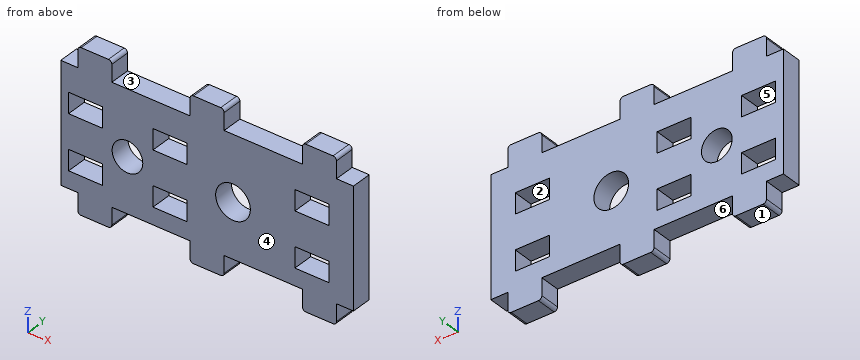
```python
from build123d import *

# Parameters (mm, degrees)
SKETCH1_W               = 86
SKETCH1_H               = 35
BOSS_EXTRUDE1_DEPTH     = 6
SKETCH2_R               = 5.1
SKETCH2_R_2             = 4.5
CUT_EXTRUDE1_DEPTH      = 6
SKETCH234_W             = 10
SKETCH234_H             = 6
BOSS_EXTRUDE234_DEPTH   = 6
FILLET134_R             = 1
SKETCH2341_W            = 10
SKETCH2341_H            = 6
BOSS_EXTRUDE2341_DEPTH  = 6
FILLET1341_R            = 1
SKETCH2342_W            = 10
SKETCH2342_H            = 6
BOSS_EXTRUDE2342_DEPTH  = 6
FILLET1342_R            = 1
FILLET134_OF_MIRROR1_R  = 1
FILLET1341_OF_MIRROR1_R = 1
FILLET1342_OF_MIRROR1_R = 1
SKETCH6_W               = 10
SKETCH6_H               = 6
CUT_EXTRUDE11_DEPTH     = 4
SKETCH61_W              = 10
SKETCH61_H              = 6
CUT_EXTRUDE12_DEPTH     = 4
SKETCH62_W              = 10
SKETCH62_H              = 6
CUT_EXTRUDE13_DEPTH     = 4


with BuildPart() as part:
    # Sketch1 → Boss-Extrude1 (new body)
    with BuildSketch(Plane(origin=(0, 0, 0), x_dir=(1, 0, 0), z_dir=(0, 1, 0))):
        with Locations((43, 17.5)):
            Rectangle(SKETCH1_W, SKETCH1_H)
    extrude(amount=BOSS_EXTRUDE1_DEPTH)

    # Sketch2 → Cut-Extrude1 (cut)
    with BuildSketch(Plane(origin=(0, 6, 0), x_dir=(1, 0, 0), z_dir=(0, 1, 0))):
        with Locations((50.6, 19)):
            Circle(SKETCH2_R)
        with Locations((19.6, 19)):
            Circle(SKETCH2_R_2)
    extrude(amount=-CUT_EXTRUDE1_DEPTH, mode=Mode.SUBTRACT)

    # Sketch234 → Boss-Extrude234 (add)
    with BuildSketch(Plane(origin=(9.232221392, 0, 0), x_dir=(1, 0, 0), z_dir=(0, 0, 1))):
        with Locations((0.767778608, 3)):
            Rectangle(SKETCH234_W, SKETCH234_H)
    boss_extrude234 = extrude(amount=BOSS_EXTRUDE234_DEPTH)

    # Fillet134
    fillet134_edges = [part.edges().sort_by_distance(p)[0] for p in [
        (5, 3, 6),
        (15, 3, 6),
    ]]
    fillet(fillet134_edges, radius=FILLET134_R)

    # Sketch2341 → Boss-Extrude2341 (add)
    with BuildSketch(Plane(origin=(42.232221392, 0, 0), x_dir=(1, 0, 0), z_dir=(0, 0, 1))):
        with Locations((0.767778608, 3)):
            Rectangle(SKETCH2341_W, SKETCH2341_H)
    boss_extrude2341 = extrude(amount=BOSS_EXTRUDE2341_DEPTH)

    # Fillet1341
    fillet1341_edges = [part.edges().sort_by_distance(p)[0] for p in [
        (48, 3, 6),
        (38, 3, 6),
    ]]
    fillet(fillet1341_edges, radius=FILLET1341_R)

    # Sketch2342 → Boss-Extrude2342 (add)
    with BuildSketch(Plane(origin=(75.232221392, 0, 0), x_dir=(1, 0, 0), z_dir=(0, 0, 1))):
        with Locations((0.767778608, 3)):
            Rectangle(SKETCH2342_W, SKETCH2342_H)
    boss_extrude2342 = extrude(amount=BOSS_EXTRUDE2342_DEPTH)

    # Fillet1342
    fillet1342_edges = [part.edges().sort_by_distance(p)[0] for p in [
        (81, 3, 6),
        (71, 3, 6),
    ]]
    fillet(fillet1342_edges, radius=FILLET1342_R)

    # Mirror1: Boss-Extrude234, Boss-Extrude2341, Boss-Extrude2342 across plane
    add(boss_extrude234.mirror(Plane(origin=(0, 0, -17.5), x_dir=(1, 0, 0), z_dir=(0, 0, -1))))
    add(boss_extrude2341.mirror(Plane(origin=(0, 0, -17.5), x_dir=(1, 0, 0), z_dir=(0, 0, -1))))
    add(boss_extrude2342.mirror(Plane(origin=(0, 0, -17.5), x_dir=(1, 0, 0), z_dir=(0, 0, -1))))

    # Fillet134 of Mirror1
    fillet134_of_mirror1_edges = [part.edges().sort_by_distance(p)[0] for p in [
        (5, 3, -41),
        (15, 3, -41),
    ]]
    fillet(fillet134_of_mirror1_edges, radius=FILLET134_OF_MIRROR1_R)

    # Fillet1341 of Mirror1
    fillet1341_of_mirror1_edges = [part.edges().sort_by_distance(p)[0] for p in [
        (48, 3, -41),
        (38, 3, -41),
    ]]
    fillet(fillet1341_of_mirror1_edges, radius=FILLET1341_OF_MIRROR1_R)

    # Fillet1342 of Mirror1
    fillet1342_of_mirror1_edges = [part.edges().sort_by_distance(p)[0] for p in [
        (81, 3, -41),
        (71, 3, -41),
    ]]
    fillet(fillet1342_of_mirror1_edges, radius=FILLET1342_OF_MIRROR1_R)

    # Sketch6 → Cut-Extrude11 (cut, symmetric)
    with BuildSketch(Plane(origin=(73.032221392, 3, -55), x_dir=(1, 0, 0), z_dir=(0, 1, 0))):
        with Locations((0.767778608, -44)):
            Rectangle(SKETCH6_W, SKETCH6_H)
    cut_extrude11 = extrude(amount=CUT_EXTRUDE11_DEPTH, both=True, mode=Mode.SUBTRACT)

    # Sketch61 → Cut-Extrude12 (cut, symmetric)
    with BuildSketch(Plane(origin=(31.332221392, 3, -55), x_dir=(1, 0, 0), z_dir=(0, 1, 0))):
        with Locations((0.767778608, -44)):
            Rectangle(SKETCH61_W, SKETCH61_H)
    cut_extrude12 = extrude(amount=CUT_EXTRUDE12_DEPTH, both=True, mode=Mode.SUBTRACT)

    # Sketch62 → Cut-Extrude13 (cut, symmetric)
    with BuildSketch(Plane(origin=(6.532221392, 3, -55), x_dir=(1, 0, 0), z_dir=(0, 1, 0))):
        with Locations((0.767778608, -44)):
            Rectangle(SKETCH62_W, SKETCH62_H)
    cut_extrude13 = extrude(amount=CUT_EXTRUDE13_DEPTH, both=True, mode=Mode.SUBTRACT)

    # Mirror2: Cut-Extrude11, Cut-Extrude12, Cut-Extrude13 across plane
    add(cut_extrude11.mirror(Plane(origin=(0, 0, -19), x_dir=(1, 0, 0), z_dir=(0, 0, -1))), mode=Mode.SUBTRACT)
    add(cut_extrude12.mirror(Plane(origin=(0, 0, -19), x_dir=(1, 0, 0), z_dir=(0, 0, -1))), mode=Mode.SUBTRACT)
    add(cut_extrude13.mirror(Plane(origin=(0, 0, -19), x_dir=(1, 0, 0), z_dir=(0, 0, -1))), mode=Mode.SUBTRACT)


solid = part.part
```
Could you check a few things on this model? Use its own coordinates, in mm. Face numbers are marked on the shaded views. A direction names the side the tool comes from. Coordinates: 2 decimals unless noted, no trailing zeros. Loops run counter-clockwise (first coordinate to the right, second up) from the corner with the lowest first, then second, coordinate; pieces in that order, holes last. Notation, with made-up numbers: M 77,71 L 130,71 A17 ccw 130,80 Z; hole C 80.5,88.5 d2. An arc over 180 degrees is marked long. Put each result on its own line as item: value. Start each with the question number.
(1) Suppose I cut it at D-D on x = 32.5. Please give me the cut outline in (y, z), then the cut area to 3 significant figures.
(2) For the marked faces 3, 4, 5 and 6, which set-ups out of +Z, -Z, +X, -X, +Y, -Y let a thin tool reach every point of the face, with its end or its side?
(3) Suppose I cut it at C-C on z = -9.5. Please give me the cut outline in (x, y), then the cut area to 3 significant figures.
(4) Suppose I cut it at B-B on z = -38. Please give me the cut outline in (x, y).
(5) Suppose I cut it at A-A on x = 19.6. Please give me the cut outline in (y, z).
(6) I need wall thicknesses on line 1 (Z direction, x = 70, y = 5); line 2 (X direction, y = 4.15, z = -13); line 3 (X direction, y = 2.15, z = -19). Which ranges of each line are inside material? Lowest first, please. Write a range as from..to.
(7) Thinking about a two-plate mould opening in X: for the marked faces 1 and 2, which applies, pulls with the +X half, pulls with the -X half, needs draft (parallel to the pull), parting line crosses it, or undercut?
(8) Will these pins go through, and if not, where does the flat tip stop? P1, Ø3, axis at x = 50.5, y = 2, coming from the -Z side; P2, Ø1.5, axis at y = 4, z = 2.5, coming from the -X side; P3, Ø3, axis at y = 3, z = -2, coming from the -X side; P4, Ø1.5, axis at x = 1.5, y = 2.5, coming from the +Z side.
Solutions:
1. outline: M 0,-35 L 6,-35 L 6,-30 L 0,-30 Z; M 0,-24 L 6,-24 L 6,-14 L 0,-14 Z; M 0,-8 L 6,-8 L 6,0 L 0,0 Z
1. area: 138 mm2
2. face 3: +Z, +Y, -Y
2. face 4: +Z, -Z, +X, -X, -Y
2. face 5: +Y, -Y
2. face 6: -Z, +Y, -Y
3. outline: M 0,0 L 2.3,0 L 2.3,6 L 0,6 Z; M 12.3,0 L 27.1,0 L 27.1,6 L 12.3,6 Z; M 37.1,0 L 68.8,0 L 68.8,6 L 37.1,6 Z; M 78.8,0 L 86,0 L 86,6 L 78.8,6 Z
3. area: 336 mm2
4. outline: M 5,0 L 15,0 L 15,6 L 5,6 Z; M 38,0 L 48,0 L 48,6 L 38,6 Z; M 71,0 L 81,0 L 81,6 L 71,6 Z
5. outline: M 0,-35 L 6,-35 L 6,-23.5 L 0,-23.5 Z; M 0,-14.5 L 6,-14.5 L 6,0 L 0,0 Z
6. line 1: z = -35..-30, -24..-14, -8..0
6. line 2: x = 0..2.3, 12.3..27.1, 37.1..68.8, 78.8..86
6. line 3: x = 0..15.1, 24.1..45.5, 55.7..86
7. face 1: needs draft
7. face 2: undercut
8. P1: stops at z = -35
8. P2: stops at x = 5
8. P3: stops at x = 0
8. P4: stops at z = 0
